Geometry: see drawing. Coordinates: mm, zero at the bounding-box minimum. Give positions to 0.01 mm unless a question says otherwise; leave off trailing zeros. Write each loop counter-clockwise with the first axis right and the second up, starting at its lowest first coordinate (ties: lowest second). Pieces come first, ordered by that corner, then holes. Notation, with made-up numbers: (30, 34) -> (58, 34) arc R18 ccw to (58, 60) -> close; hole circle Ø2 at (13, 47.5). An arc over 180 degrees is marked (long way). Use CSV: the item, a comma, the result in double quotes. Start each with the question number.
1) Section D-D (y = 23.5). Output: boundary loops of the cut face in (x, z).
2) Material intervals for line 1 (Z direction, x = 20.32, y = 17); line 2 (Y direction, x = 55, z = 27); line 3 (Y direction, x = 55.5, z = 16), sorted ascending. Write a range as [from, to].
3) Section A-A (y = 17). Output: boundary loops of the cut face in (x, z), plus the area to 3 significant figures.
4) Section C-C (x = 20.32). Output: boundary loops of the cut face in (y, z).
5) Draft query along Z for the marked faces 1, 2, 3 and 4. Return one class per face: pulls with the +Z half, pulls with the -Z half, needs draft (parallel to the pull), parting line crosses it, or undercut.
6) Section B-B (z = 35.56). Output: boundary loops of the cut face in (x, y).
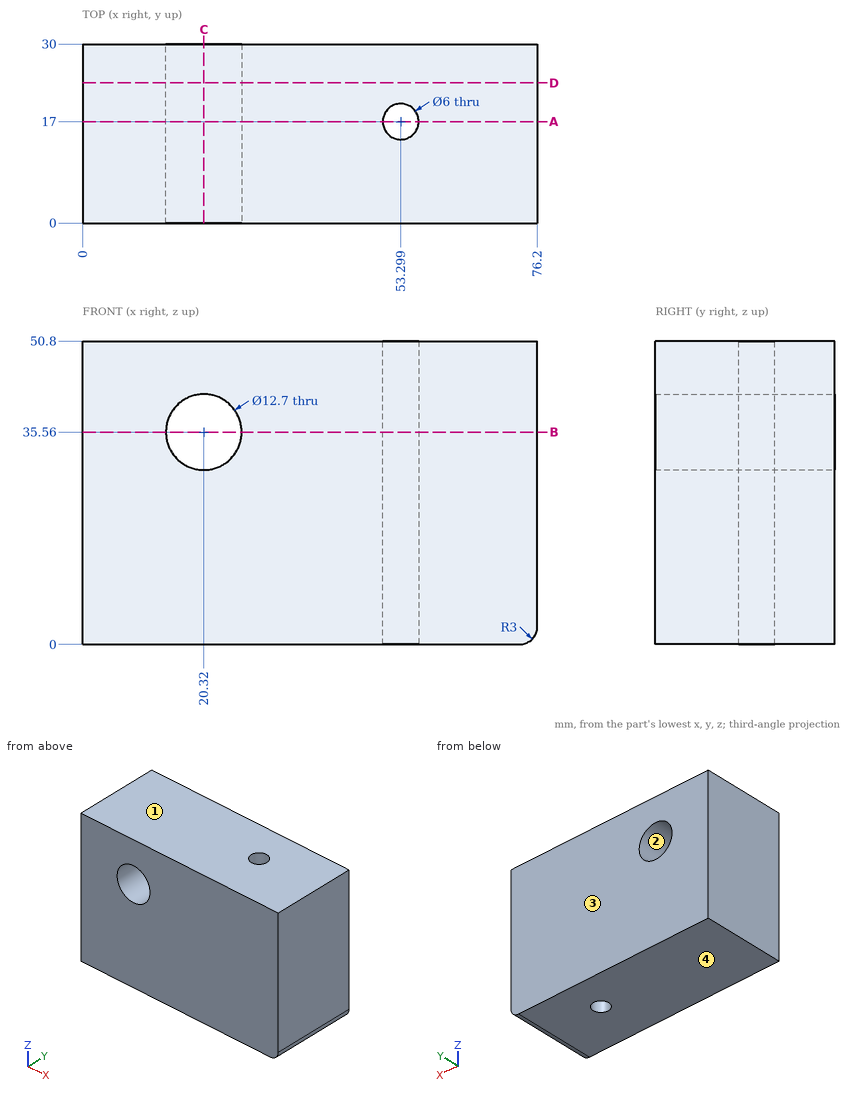
Answers follow:
1,outline,"(0, 0) -> (73.2, 0) arc R3 ccw to (76.2, 3) -> (76.2, 50.8) -> (0, 50.8) -> close; hole circle Ø12.7 at (20.32, 35.56)"
2,line 1,"z = [0, 29.21], [41.91, 50.8]"
2,line 2,"y = [0, 14.53], [19.47, 30]"
2,line 3,"y = [0, 14.96], [19.04, 30]"
3,outline,"(0, 0) -> (50.3, 0) -> (50.3, 50.8) -> (0, 50.8) -> close; (56.3, 0) -> (73.2, 0) arc R3 ccw to (76.2, 3) -> (76.2, 50.8) -> (56.3, 50.8) -> close; hole circle Ø12.7 at (20.32, 35.56)"
3,area,"3,440 mm^2"
4,outline,"(0, 0) -> (30, 0) -> (30, 29.21) -> (0, 29.21) -> close; (0, 41.91) -> (30, 41.91) -> (30, 50.8) -> (0, 50.8) -> close"
5,face 1,"pulls with the +Z half"
5,face 2,"undercut"
5,face 3,"needs draft"
5,face 4,"pulls with the -Z half"
6,outline,"(0, 0) -> (13.97, 0) -> (13.97, 30) -> (0, 30) -> close; (26.67, 0) -> (76.2, 0) -> (76.2, 30) -> (26.67, 30) -> close; hole circle Ø6 at (53.3, 17)"
